```python
from build123d import *

# Parameters (mm, degrees)
SKETCH_1_R          = 15
EXTRUDE_1_DEPTH     = 2.3
SKETCH_2_R          = 1.5
CUT_EXTRUDE_1_DEPTH = 2.3
EXTRUDE_2_DEPTH     = 4.6
CUT_EXTRUDE_2_DEPTH = 3.7
CUT_EXTRUDE_START   = -2.3
CUT_EXTRUDE_3_DEPTH = 2.3
FILLET_1_R          = 1
SKETCH_6_R          = 7.45
EXTRUDE_3_DEPTH     = 4.4
SKETCH_7_R          = 6.25
EXTRUDE_4_DEPTH     = 6
SKETCH_8_R          = 5.5
CUT_EXTRUDE_4_DEPTH = 4
SKETCH_9_R          = 4.5
CUT_EXTRUDE_5_DEPTH = 25.724279565
CUT_EXTRUDE_START_2 = -4
SKETCH_10_R         = 5.5
CUT_EXTRUDE_6_DEPTH = 4
CHAMFER_1_SIZE      = 0.05
FILLET_2_R          = 0.5


with BuildPart() as part:
    # Эскиз1 → Бобышка-Вытянуть1 (new body)
    with BuildSketch(Plane(origin=(0, 0, 0), x_dir=(1, 0, 0), z_dir=(0, 1, 0))):
        with Locations(Location((0, 0, 0), (0, 0, 270))):
            Circle(SKETCH_1_R)
    extrude(amount=EXTRUDE_1_DEPTH)

    # Эскиз2 → Вырез-Вытянуть1 (cut)
    with BuildSketch(Plane.XZ):
        with BuildLine():
            ThreePointArc((-10.419812858, 2.5), (-12.091025454, 3.401342429), (-12.25590323, 5.292951542))
            ThreePointArc((-12.25590323, 5.292951542), (-9.439875529, 9.439875529), (-5.292951542, 12.25590323))
            ThreePointArc((-5.292951542, 12.25590323), (-3.401342429, 12.091025454), (-2.5, 10.419812858))
            Line((-2.5, 10.419812858), (-2.5, 8.366600265))
            ThreePointArc((-2.5, 8.366600265), (-2.783209849, 7.340621913), (-3.552631579, 6.605210736))
            ThreePointArc((-3.552631579, 6.605210736), (-5.303300859, 5.303300859), (-6.605210736, 3.552631579))
            ThreePointArc((-6.605210736, 3.552631579), (-7.340621913, 2.783209849), (-8.366600265, 2.5))
            Line((-8.366600265, 2.5), (-10.419812858, 2.5))
        make_face()
        with Locations(Location((0, 9.5, 0), (0, 0, 270))):
            Circle(SKETCH_2_R)
        with BuildLine():
            ThreePointArc((2.5, 10.419812858), (3.401342429, 12.091025454), (5.292951542, 12.25590323))
            ThreePointArc((5.292951542, 12.25590323), (9.439875529, 9.439875529), (12.25590323, 5.292951542))
            ThreePointArc((12.25590323, 5.292951542), (12.091025454, 3.401342429), (10.419812858, 2.5))
            Line((10.419812858, 2.5), (8.366600265, 2.5))
            ThreePointArc((8.366600265, 2.5), (7.340621913, 2.783209849), (6.605210736, 3.552631579))
            ThreePointArc((6.605210736, 3.552631579), (5.303300859, 5.303300859), (3.552631579, 6.605210736))
            ThreePointArc((3.552631579, 6.605210736), (2.783209849, 7.340621913), (2.5, 8.366600265))
            Line((2.5, 8.366600265), (2.5, 10.419812858))
        make_face()
        with Locations(Location((12.5, 0, 0), (0, 0, 270))):
            Circle(SKETCH_2_R)
        with BuildLine():
            ThreePointArc((10.419812858, -2.5), (12.091025454, -3.401342429), (12.25590323, -5.292951542))
            ThreePointArc((12.25590323, -5.292951542), (9.439875529, -9.439875529), (5.292951542, -12.25590323))
            ThreePointArc((5.292951542, -12.25590323), (3.401342429, -12.091025454), (2.5, -10.419812858))
            Line((2.5, -10.419812858), (2.5, -8.366600265))
            ThreePointArc((2.5, -8.366600265), (2.783209849, -7.340621913), (3.552631579, -6.605210736))
            ThreePointArc((3.552631579, -6.605210736), (5.303300859, -5.303300859), (6.605210736, -3.552631579))
            ThreePointArc((6.605210736, -3.552631579), (7.340621913, -2.783209849), (8.366600265, -2.5))
            Line((8.366600265, -2.5), (10.419812858, -2.5))
        make_face()
        with Locations(Location((0, -9.5, 0), (0, 0, 270))):
            Circle(SKETCH_2_R)
        with BuildLine():
            ThreePointArc((-2.5, -10.419812858), (-3.401342429, -12.091025454), (-5.292951542, -12.25590323))
            ThreePointArc((-5.292951542, -12.25590323), (-9.439875529, -9.439875529), (-12.25590323, -5.292951542))
            ThreePointArc((-12.25590323, -5.292951542), (-12.091025454, -3.401342429), (-10.419812858, -2.5))
            Line((-10.419812858, -2.5), (-8.366600265, -2.5))
            ThreePointArc((-8.366600265, -2.5), (-7.340621913, -2.783209849), (-6.605210736, -3.552631579))
            ThreePointArc((-6.605210736, -3.552631579), (-5.303300859, -5.303300859), (-3.552631579, -6.605210736))
            ThreePointArc((-3.552631579, -6.605210736), (-2.783209849, -7.340621913), (-2.5, -8.366600265))
            Line((-2.5, -8.366600265), (-2.5, -10.419812858))
        make_face()
        with Locations(Location((-12.5, 0, 0), (0, 0, 270))):
            Circle(SKETCH_2_R)
    extrude(amount=-CUT_EXTRUDE_1_DEPTH, mode=Mode.SUBTRACT)

    # Эскиз3 → Бобышка-Вытянуть2 (add)
    with BuildSketch(Plane.XZ):
        with BuildLine():
            Line((-5.476192266, 10.284518378), (-7.9263742, 12.734700312))
            ThreePointArc((-7.9263742, 12.734700312), (-10.606601718, 10.606601718), (-12.734700312, 7.9263742))
            Line((-12.734700312, 7.9263742), (-10.284518378, 5.476192266))
            ThreePointArc((-10.284518378, 5.476192266), (-9.471553651, 5.188917785), (-8.737287773, 5.640904394))
            ThreePointArc((-8.737287773, 5.640904394), (-7.353910524, 7.353910524), (-5.640904394, 8.737287773))
            ThreePointArc((-5.640904394, 8.737287773), (-5.188917785, 9.471553651), (-5.476192266, 10.284518378))
        make_face()
    extrude(amount=-EXTRUDE_2_DEPTH)

    # Эскиз4 → Вырез-Вытянуть2 (cut)
    with BuildSketch(Plane.XZ):
        with BuildLine():
            Line((-7.609089602, 10.437516727), (-11.362124092, 14.190551216))
            Line((-11.362124092, 14.190551216), (-14.190551216, 11.362124092))
            Line((-14.190551216, 11.362124092), (-10.437516727, 7.609089602))
            ThreePointArc((-10.437516727, 7.609089602), (-9.691317564, 7.316960783), (-8.970221669, 7.666493541))
            ThreePointArc((-8.970221669, 7.666493541), (-8.343860018, 8.343860018), (-7.666493541, 8.970221669))
            ThreePointArc((-7.666493541, 8.970221669), (-7.316960783, 9.691317564), (-7.609089602, 10.437516727))
        make_face()
    extrude(amount=-CUT_EXTRUDE_2_DEPTH, mode=Mode.SUBTRACT)

    # Эскиз5 → Вырез-Вытянуть3 (cut)
    with BuildSketch(Plane(origin=(0, 4.6, 0), x_dir=(1, 0, 0), z_dir=(0, 1, 0)).offset(CUT_EXTRUDE_START)):
        with BuildLine():
            Line((-12.937905898, -5.348886891), (-9.109525824, -3.766129051))
            Line((-9.109525824, -3.766129051), (-3.979530291, -8.038651188))
            Line((-3.979530291, -8.038651188), (-5.138314359, -13.022969152))
            ThreePointArc((-5.138314359, -13.022969152), (-9.818875666, -9.979462944), (-12.937905898, -5.348886891))
        make_face()
    extrude(amount=CUT_EXTRUDE_3_DEPTH, mode=Mode.SUBTRACT)

    # Скругление1
    fillet_1_edges = [part.edges().sort_by_distance(p)[0] for p in [
        (-11.532758238, 1.15, 6.724432126),
        (-6.724432126, 1.15, 11.532758238),
    ]]
    fillet(fillet_1_edges, radius=FILLET_1_R)

    # Эскиз6 → Бобышка-Вытянуть3 (add)
    with BuildSketch(Plane(origin=(0, 2.3, 0), x_dir=(1, 0, 0), z_dir=(0, 1, 0))):
        with Locations(Location((0, 0, 0), (0, 0, 270))):
            Circle(SKETCH_6_R)
    extrude(amount=EXTRUDE_3_DEPTH)

    # Эскиз7 → Бобышка-Вытянуть4 (add)
    with BuildSketch(Plane(origin=(0, 6.7, 0), x_dir=(1, 0, 0), z_dir=(0, 1, 0))):
        with Locations(Location((0, 0, 0), (0, 0, 270))):
            Circle(SKETCH_7_R)
    extrude(amount=EXTRUDE_4_DEPTH)

    # Эскиз8 → Вырез-Вытянуть4 (cut)
    with BuildSketch(Plane(origin=(0, 12.7, 0), x_dir=(1, 0, 0), z_dir=(0, 1, 0))):
        with Locations(Location((0, 0, 0), (0, 0, 270))):
            Circle(SKETCH_8_R)
    extrude(amount=-CUT_EXTRUDE_4_DEPTH, mode=Mode.SUBTRACT)

    # Эскиз9 → Вырез-Вытянуть5 (cut, through all)
    with BuildSketch(Plane.XZ):
        with Locations(Location((0, 0, 0), (0, 0, 270))):
            Circle(SKETCH_9_R)
    extrude(amount=-CUT_EXTRUDE_5_DEPTH, mode=Mode.SUBTRACT)

    # Эскиз10 → Вырез-Вытянуть6 (cut)
    with BuildSketch(Plane.XZ.offset(CUT_EXTRUDE_START_2)):
        with Locations(Location((0, 0, 0), (0, 0, 90))):
            Circle(SKETCH_10_R)
    extrude(amount=CUT_EXTRUDE_6_DEPTH, mode=Mode.SUBTRACT)

    # Фаска1
    chamfer_1_edges = [part.edges().sort_by_distance(p)[0] for p in [
        (-5.615881331, 0, 10.424207443),
        (-9.471553651, 0, 5.188917785),
        (-7.353910524, 0, 7.353910524),
        (-5.188917785, 0, 9.471553651),
        (-11.181814155, 0, 8.35338703),
        (-9.691317564, 0, 7.316960783),
        (-8.343860018, 0, 8.343860018),
        (-7.316960783, 0, 9.691317564),
        (-8.35338703, 0, 11.181814155),
        (-12.220045296, 0, 5.375220272),
        (-10.424207443, 0, 5.615881331),
        (-6.03192206, 0, 11.452137177),
        (-11.452137177, 0, 6.03192206),
        (0, 12.7, -6.25),
        (0, 12.7, -5.5),
        (0, 0, -5.5),
        (3.401342429, 0, 12.091025454),
        (7.340621913, 0, 2.783209849),
        (5.303300859, 0, 5.303300859),
        (2.5, 0, 9.393206562),
        (2.783209849, 0, 7.340621913),
        (9.393206562, 0, 2.5),
        (12.091025454, 0, 3.401342429),
        (9.439875529, 0, 9.439875529),
        (12.091025454, 0, -3.401342429),
        (2.5, 0, -9.393206562),
        (2.783209849, 0, -7.340621913),
        (5.303300859, 0, -5.303300859),
        (9.393206562, 0, -2.5),
        (7.340621913, 0, -2.783209849),
        (3.401342429, 0, -12.091025454),
        (9.439875529, 0, -9.439875529),
        (-3.401342429, 0, -12.091025454),
        (-9.393206562, 0, -2.5),
        (-7.340621913, 0, -2.783209849),
        (-5.303300859, 0, -5.303300859),
        (-2.5, 0, -9.393206562),
        (-2.783209849, 0, -7.340621913),
        (-12.091025454, 0, -3.401342429),
        (-9.439875529, 0, -9.439875529),
        (-12.091025454, 0, 3.401342429),
        (-2.783209849, 0, 7.340621913),
        (-5.303300859, 0, 5.303300859),
        (-9.393206562, 0, 2.5),
        (-7.340621913, 0, 2.783209849),
        (-2.5, 0, 9.393206562),
        (-3.401342429, 0, 12.091025454),
        (-5.375220272, 0, 12.220045296),
    ]]
    chamfer(chamfer_1_edges, length=CHAMFER_1_SIZE)

    # Скругление2
    fillet_2_edges = [part.edges().sort_by_distance(p)[0] for p in [
        (-7.9263742, 3.45, 12.734700312),
        (-7.198961436, 3.45, 12.007287548),
        (-12.734700312, 3.45, 7.9263742),
        (-12.007287548, 3.45, 7.198961436),
    ]]
    fillet(fillet_2_edges, radius=FILLET_2_R - 0.0001)  # a hair under: the kernel refuses the full size


solid = part.part
```
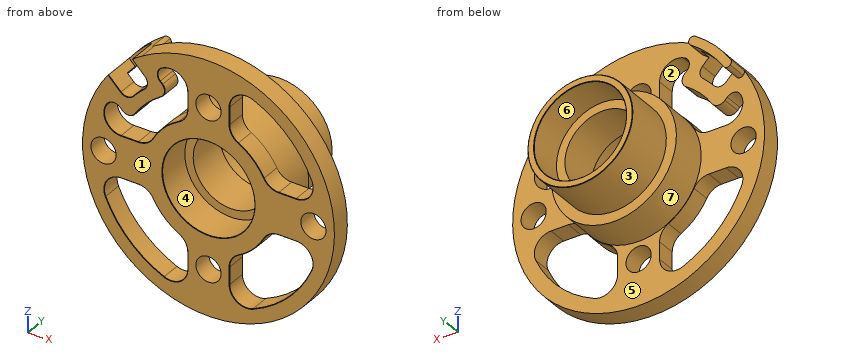
Here's how the part is built. I have some questions about the finished solid (model axes, mm). Face numbers are marked on the shaded views. A direction names the side the tool comes from. Round coordinates to 2 decimals unless told otherwise and drop trailing zeros. Order: outer loops, then holes, each group sorted by start corner. A loop starts at its lowest first (then second) coordinate and runs counter-clockwise, first axis right, second up. Notation, with made-up numbers: (86.25, -11) -> (142.25, -11) arc R26 ccw to (142.25, 8) -> close; hole circle Ø1 at (-16, 60.25). An arc over 180 degrees is marked (long way). Use a Markdown table: item, result. Add a question column.
(1) If we mould it in two halves opening along Z, with no side actions, what happens to the marked faces 4, 5, 6 and 7? For each: released by +Z, released by -Z, zero draft, split by the parting line, or undercut.
(2) Suppose I cut it at C-C, the plane z = 0. Count the separate pieces of the cut face and the enclosed holes in it, and give its area (3 significant figures).
(3) For pin 1 Ø1 at (y, z) = (1.5, 9) entering from -X; pin 2 Ø1 at (y, z) = (1, -9) entering from +X; pin 3 Ø3 at (x, y) = (6, 7) entering from +Z, each with a flat end and sliding along its axis, tell me the tip position at first contact or that it passes through.
(4) I need wall thicknesses on line 1 along X through (y, z) = (11.35, 0); line 2 along Z through (x, y) = (-0.75, 1.5); line 3 along X through (y, z) = (3.1, 0). Which ranges of each line are inside material? Lowest first, please.
(5) For the marked faces 1, 2 and 3, which set-ups out of +Z, -Z, +X, -X, +Y, -Y let a thin tool reach every point of the face, with its end or its side?
(6) Suppose I cut it at A-A, the plane y = 10.5. Please give me the cut outline in (x, z), and give its area (3 significant figures).
(7) Suppose I cut it at B-B, the plane x = 13. Please give me the cut outline in (y, z), and give its area (3 significant figures).
Verdict:
| question | item | result |
|---|---|---|
| 1 | face 4 | undercut |
| 1 | face 5 | zero draft |
| 1 | face 6 | undercut |
| 1 | face 7 | split by the parting line |
| 2 | separate pieces | 4 |
| 2 | enclosed holes | 0 |
| 2 | area | 65.5 mm2 |
| 3 | pin 1 | x = -12.36 |
| 3 | pin 2 | x = 12.36 |
| 3 | pin 3 | z = 5.91 |
| 4 | line 1 | -6.25 to -5.5, 5.5 to 6.25 |
| 4 | line 2 | -14.98 to -10.8, -8.2 to -5.45, 5.45 to 8.2, 10.8 to 14.98 |
| 4 | line 3 | -7.45 to -5.5, 5.5 to 7.45 |
| 5 | face 1 | +Z, -Z, +X, -X, -Y |
| 5 | face 2 | +Y, -Y |
| 5 | face 3 | +Y |
| 6 | outline | circle Ø12.5 at (0, 0); hole circle Ø11 at (0, 0) |
| 6 | area | 27.7 mm2 |
| 7 | outline | (0, -7.48) -> (2.3, -7.48) -> (2.3, -1.41) -> (0, -1.41) -> close; (0, 1.41) -> (2.3, 1.41) -> (2.3, 7.48) -> (0, 7.48) -> close |
| 7 | area | 27.9 mm2 |
